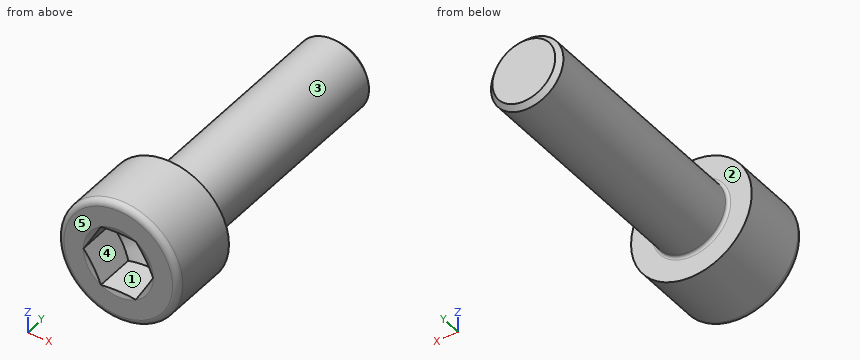
Solid Edge part; units mm, degrees
sketch "Sketch1" plane through (0, 0, 0) normal (0, 0, 1) x (1, 0, 0)
  line L0 (3, 0) -> (3, 20)
  line L1 (0, 20) -> (3, 20)
  line L2 (0, 0) -> (0, 20)
  line L3 (0, 0) -> (0, -6)
  line L4 (0, -6) -> (5, -6)
  line L5 (5, -6) -> (5, 0)
  line L6 (5, 0) -> (3, 0)
revolve "RevolvedProtrusion1" add sketch "Sketch1" angle 360 about axis through (0, 0, 0) along (0, 1, 0)
sketch "Sketch2" plane through (0, 0, 0) normal (1, 0, 0) x (0, 1, 0)
  line L0 (-6, 3.3615) -> (-3, 3.3615)
  line L1 (-1.0592, 0) -> (-3, 3.3615)
  line L2 (-6, 0) -> (-1.0592, 0)
  line L3 (-6, 0) -> (-6, 3.3615)
revolve "RevolvedCutout1" cut sketch "Sketch2" angle 360 about axis through (0, -4.5, 0) along (0, 1, 0)
sketch "Sketch3" plane through (0, -6, 0) normal (0, -1, 0) x (0, 0, 1)
  circle A0 centre (0, 0) radius 3.3615
  line L0 (-2.5, -1.4434) -> (0, -2.8868)
  line L1 (0, -2.8868) -> (2.5, -1.4434)
  line L2 (2.5, -1.4434) -> (2.5, 1.4434)
  line L3 (2.5, 1.4434) -> (0, 2.8868)
  line L4 (0, 2.8868) -> (-2.5, 1.4434)
  line L5 (-2.5, 1.4434) -> (-2.5, -1.4434)
extrude "Protrusion1" add sketch "Sketch3" against normal up to next
sketch "Sketch4" plane through (0, 0, 0) normal (0, 0, 1) x (1, 0, 0)
  line L0 (-2.8868, -6) -> (0, -6)
  line L1 (0, -6) -> (0, -5.2265)
  line L2 (0, -5.2265) -> (-2.8868, -6)
revolve "RevolvedCutout2" cut sketch "Sketch4" angle 360 about axis through (0, -4.5, 0) along (0, 1, 0)
fillet "Round1" radius 0.25 1 edges at (0, 0, -3)
fillet "Round2" radius 0.5 1 edges at (0, -6, -5)
chamfer "倒斜角_2" distance 0.4 angle 45 1 edges at (0, 20, -3)
cosmetic_thread "螺纹_3" thread depth 16
Part model, mm, in its own coordinate system. Face numbers are marked on the shaded views. A direction names the side the tool comes from. Round coordinates to 2 decimals unless told otherwise and drop trailing zeros. Write each loop counter-clockwise with the first axis right and the second up, starting at its lowest first coordinate (ties: lowest second). Pieces come first, ordered by that corner, then holes. Notation, with made-up numbers: (-2.75, 31.5) -> (47.25, 31.5) arc R32 cw to (47.25, 59.5) -> close; hole circle Ø1 at (-18, 51.25). An arc over 180 degrees is marked (long way). Return JSON: item names as keys, results as strings. Group by question number.
Q1. Probe L1, parallel to Y at x = -3.5, z = -1.5; L2, parallel to X at y = 13, z = -1.5. List the from-to ranges inside material, lowest first. Write a range as [from, to].
Q2. Which spindle directions (+Z, -Z, +X, -X, +Y, -Y) get a long thin tool onto all of the face, cutting with end or side? Do the marked faces 4 and 5. Say none if no direction does.
Q3. Mould opens along Z. For the marked faces 1, 2 and 3 say: pulls with the +Z half, pulls with the -Z half, needs draft (parallel to the pull), parting line crosses it, or undercut.
Q4. Saw through at A-A on y = 1.75. Write the cut outline in (x, z).
Q5. Pin check, flat tip, straight feed: pin 1 (5 mm diameter, centred on x = -3.5, z = 4, fed in from +Y). Stop position of the tip, or through.
Answer:
{
 "1": {"L1": "[-6, 0]", "L2": "[-2.6, 2.6]"},
 "2": {"face 4": "-Y", "face 5": "+Z, -Z, +X, -X, -Y"},
 "3": {"face 1": "undercut", "face 2": "needs draft", "face 3": "parting line crosses it"},
 "4": {"outline": "circle Ø6 at (0, 0)"},
 "5": {"pin 1": "y = 19.78"}
}
